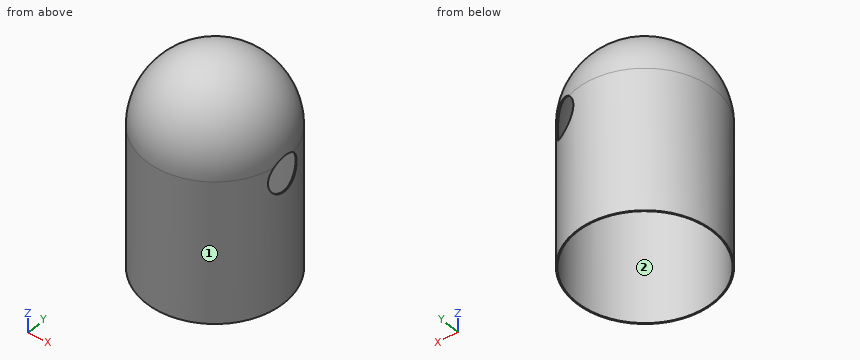
from build123d import *

# Parameters (mm, degrees)
F0_R      = 48.3
F0_R_2    = 47.5
F1_DEPTH  = 100
F3_ANGLE  = 180
F5_R      = 12.5
F6_DEPTH  = 6
F9_R      = 12.5
F10_DEPTH = 6


with BuildPart() as f1:
    # F0 (on Top) → F1 (new body)
    with BuildSketch(Plane.XY):
        Circle(F0_R)
        Circle(F0_R_2, mode=Mode.SUBTRACT)
    extrude(amount=F1_DEPTH)

    # F2 (on face) → F3 (revolve)
    with BuildSketch(Plane.XY.offset(100)):
        with BuildLine():
            ThreePointArc((47.5, 0), (0, -47.5), (-47.5, 0))
            Line((-47.5, 0), (-48.3, 0))
            ThreePointArc((-48.3, 0), (0, -48.3), (48.3, 0))
            Line((48.3, 0), (47.5, 0))
        make_face()
    revolve(axis=Axis((-47.9, 0, 100), (-1, 0, 0)), revolution_arc=F3_ANGLE)

    # F5 (on offset) → F6 (cut)
    with BuildSketch(Plane.YZ.offset(49)):
        with Locations((0, 90.8108726144)):
            Circle(F5_R)
    extrude(amount=-F6_DEPTH, mode=Mode.SUBTRACT)

    # F9 (on face) → F10 (cut)
    with BuildSketch(Plane(origin=(24.5, 42.4352447854, 0), x_dir=(-0.8660254038, 0.5, 0), z_dir=(0.5, 0.8660254038, 0))):
        with Locations((0, 90.4301926494)):
            Circle(F9_R)
    extrude(amount=-F10_DEPTH, mode=Mode.SUBTRACT)


solid = f1.part
Geometry: final body of the model. Coordinates: model frame, mm. Face numbers are marked on the shaded views. Round coordinates to 2 decimals unless told otherwise and drop trailing zeros. Loops run counter-clockwise (first coordinate to the right, second up) from the corner with the lowest first, then second, coordinate; pieces in that order, holes last. Notation, with made-up numbers: M -30,40.25 L 2,40.25 A17 cw 2,57.25 Z; hole C 72,-29 d2. An arc over 180 degrees is marked long. Put each result on its own line as item: value. Start each with the question number.
(1) Section query A-A (z = 85). Return loops of the section in (x, y).
(2) Material intervals for line 1 along Y through (x, z) = (0, 35); line 2 along X through (y, z) = (17, 34), sorted ascending. Write a range as [from, to].
(3) Contact query for flat-ended pins moving along their axis: pin 1 Ø3 at (x, y) = (17, -11) entering from +Z; pin 2 Ø2 at (x, z) = (-15, 131) entering from -Y; pin 3 Ø10 at (x, z) = (37.5, 98.5) entering from +Y. Output: stop coordinate, or through.
(4) Section query C-C (x = 0). Return loops of the section in (y, z).
(5) Draft query along Y for the marked faces 1 and 2. Return one class per face: +Y half, -Y half, draft (parallel to the pull), parting line (faces both ways), or undercut.
(6) Section query D-D (y = -27). Return loops of the section in (x, z), then the cut area to 3 significant figures.
Findings below:
1. outline: M 13.32,45.59 L 13.73,46.31 A48.3 ccw long 47.01,-11.07 L 46.19,-11.07 A47.5 cw long Z; M 32.82,34.33 A47.5 cw 46.19,11.07 L 47.01,11.07 A48.3 ccw 33.24,35.05 Z
2. line 1: y = [-48.3, -47.5], [47.5, 48.3]
2. line 2: x = [-45.21, -44.35], [44.35, 45.21]
3. pin 1: stops at z = 144.51
3. pin 2: stops at y = -34.85
3. pin 3: stops at y = 35.73
4. outline: M -48.3,0 L -47.5,0 L -47.5,100 A47.5 cw 47.5,100 L 47.5,0 L 48.3,0 L 48.3,100 A48.3 ccw -48.3,100 Z
5. face 1: parting line
5. face 2: undercut
6. outline: M -40.05,0 L -39.08,0 L -39.08,100 A39.08 cw 39.08,100 L 39.08,0 L 40.05,0 L 40.05,100 A40.05 ccw -40.05,100 Z
6. area: 314 mm2
